```python
from build123d import *

# Parameters (mm, degrees)
F0_R     = 12
F1_DEPTH = 3
F3_DEPTH = 3
F4_W     = 3
F4_H     = 3
F5_DEPTH = 3


with BuildPart() as f1:
    # F0 (on Front) → F1 (new body)
    with BuildSketch(Plane.XZ):
        with BuildLine():
            ThreePointArc((64.5, -24.5), (89, 0), (64.5, 24.5))
            Line((64.5, 24.5), (-64.5, 24.5))
            ThreePointArc((-64.5, 24.5), (-81.824116, 17.324116), (-89, 0))
            ThreePointArc((-89, 0), (-81.824116, -17.324116), (-64.5, -24.5))
            Line((-64.5, -24.5), (64.5, -24.5))
        make_face()
        with Locations((-64.5, 0)):
            Circle(F0_R, mode=Mode.SUBTRACT)
        with Locations((64.5, 0)):
            Circle(F0_R, mode=Mode.SUBTRACT)
        with BuildLine():
            ThreePointArc((-64.5, -24.5), (-81.824116, -17.324116), (-89, 0))
            Line((-89, 0), (-89, -24.5))
            Line((-89, -24.5), (-64.5, -24.5))
        make_face()
    extrude(amount=F1_DEPTH)

    # F2 (on face) → F3 (join)
    with BuildSketch(Plane.XZ.offset(3)):
        with BuildLine():
            Line((-89, 0), (-89, -24.5))
            Line((-89, -24.5), (-86, -24.5))
            Line((-86, -24.5), (-86, 0))
            ThreePointArc((-86, 0), (-79.702796, 15.202796), (-64.5, 21.5))
            Line((-64.5, 21.5), (64.5, 21.5))
            ThreePointArc((64.5, 21.5), (79.702796, 15.202796), (86, 0))
            Line((86, 0), (89, 0))
            ThreePointArc((89, 0), (81.824116, 17.324116), (64.5, 24.5))
            Line((64.5, 24.5), (-64.5, 24.5))
            ThreePointArc((-64.5, 24.5), (-81.824116, 17.324116), (-89, 0))
        make_face()
    extrude(amount=F3_DEPTH)

    # F4 (on face) → F5 (cut)
    with BuildSketch(Plane.XZ.offset(6)):
        with Locations((-87.5, -23)):
            Rectangle(F4_W, F4_H)
    extrude(amount=-F5_DEPTH, mode=Mode.SUBTRACT)


solid = f1.part
```
For this review, take the finished solid that the model builds, in its own axes (mm). A direction names the side the tool comes from. Coordinates: 2 decimals unless noted, no trailing zeros. Write each loop counter-clockwise with the first axis right and the second up, starting at its lowest first coordinate (ties: lowest second). Pieces come first, ordered by that corner, then holes.
(1) Tool access review of faces 1 (the face through (-1, -4, 21.5)), 2 (the face through (-88, -5, -21.5)), 3 (the face through (-13, -1, -24.5)), 4 (the face through (-86, -4, -11)): name each direction out of +Z, -Z, +X, -X, +Y, -Y from which nothing blocks a thin tool from reaching the whole face with its end or side.
(2) For pin 1 Ø2.5 at (x, y) = (4.5, -4) entering from -Z; pin 2 Ø0.9 at (y, z) = (-5, -10.5) entering from +X; pin 3 Ø1.5 at (x, y) = (87.5, -4) entering from -Z; pin 4 Ø14 at (x, z) = (36.5, 6.5) entering from -Y, all flat-tipped, find the tip position at first contact; note any pin that passes through.
(3) Add section B-B on z = -1.5. Give the boundary of the cut face in (x, y).
(4) Add section D-D on z = 7.5. Give the boundary of the cut face in (x, y).
(5) Wall thickness on probe 1 along Z at (x, y) = (64.5, -1.75); probe 2 along X at (y, z) = (-2.2, 10); probe 3 along X at (y, z) = (-3.3, -20): over which ranges is each line inside the solid? List them lowest first.
(6) Add section C-C on z = -19. Give the boundary of the cut face in (x, y), then the cut area to 3 significant figures.
(7) The part is to be moulded in two halves that separate along X. For faces 5 (the face through (-76.49, -1.48, 0.53)), 6 (the face through (-79.869, -4.479, 15.035)), 7 (the face through (-89, -3, -12)), 8 (the face through (-20, -6, 22)), say which applies: +X half, -X half, draft (parallel to the pull), parting line (faces both ways), or undercut.
(8) Add section A-A on y = -4.4. Give the boundary of the cut face in (x, z).
Answer sheet:
1. face 1: -Z, -Y
1. face 2: -Z, +X, -X, -Y
1. face 3: -Z, +X, -X, +Y, -Y
1. face 4: -Z, +X, -Y
2. pin 1: stops at z = -24.5
2. pin 2: stops at x = -86
2. pin 3: stops at z = 0
2. pin 4: stops at y = -3
3. outline: (-89, -6) - (-86, -6) - (-86, -3) - (-76.41, -3) - (-76.41, 0) - (-89, 0) - close; (-52.59, -3) - (52.59, -3) - (52.59, 0) - (-52.59, 0) - close; (76.41, -3) - (88.95, -3) - (88.95, 0) - (76.41, 0) - close
4. outline: (-87.82, -6) - (-84.65, -6) - (-84.65, -3) - (-73.87, -3) - (-73.87, 0) - (-87.82, 0) - close; (-55.13, -3) - (55.13, -3) - (55.13, 0) - (-55.13, 0) - close; (73.87, -3) - (84.65, -3) - (84.65, -6) - (87.82, -6) - (87.82, 0) - (73.87, 0) - close
5. probe 1: z = -24.5 to -12, 12 to 24.5
5. probe 2: x = -86.87 to -71.13, -57.87 to 57.87, 71.13 to 86.87
5. probe 3: x = -89 to -86
6. outline: (-89, -6) - (-86, -6) - (-86, -3) - (79.97, -3) - (79.97, 0) - (-89, 0) - close
6. area: 516 mm2
7. face 5: undercut
7. face 6: undercut
7. face 7: -X half
7. face 8: draft
8. outline: (-89, -21.5) - (-86, -21.5) - (-86, 0) arc R21.5 cw to (-64.5, 21.5) - (64.5, 21.5) arc R21.5 cw to (86, 0) - (89, 0) arc R24.5 ccw to (64.5, 24.5) - (-64.5, 24.5) arc R24.5 ccw to (-89, 0) - close
